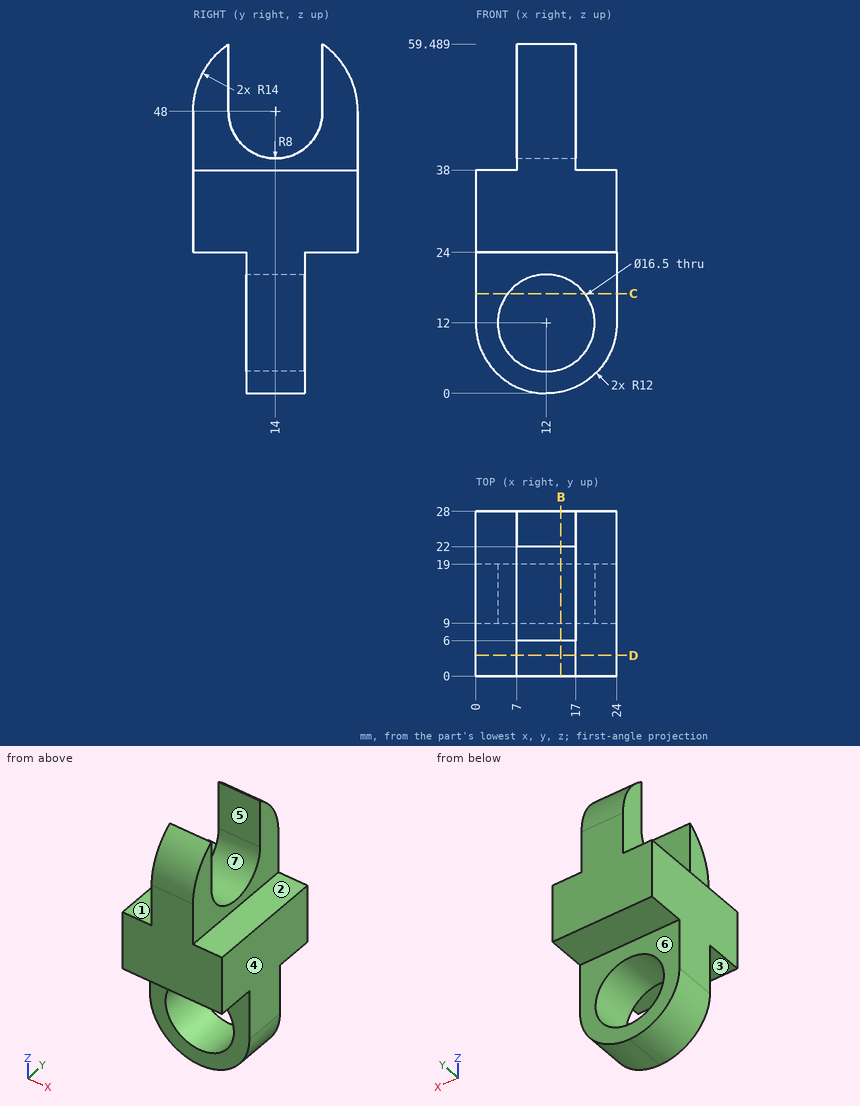
Geometry: see drawing. Coordinates: mm, zero at the bounding-box minimum. A direction names the side the tool comes from. Coordinates: 2 decimals unless noted, no trailing zeros. Loops run counter-clockwise (first coordinate to the right, second up) from the corner with the lowest first, then second, coordinate; pieces in that order, holes last. Notation, with made-up numbers: (-29, 50.25) -> (-10, 50.25) arc R13 cw to (-10, 54.25) -> close; hole circle Ø3 at (-9, 43.5). An arc over 180 degrees is marked (long way). Write item = value, one per line. Start each with the question number.
Item 1: Cut plane D-D, the plane y = 3.5. Return loops of the section in (x, z), plus the area to 3 significant figures.
Item 2: Reachability of the marked faces 1, 2 and 3 from +Z, -Z, +X, -X, +Y, -Y: full face, straight path, thin tool, end or side. Return the list, or none.
Item 3: First-contact query: P1, Ø5.5, axis at x = 3.5, y = 10.5, coming from the +Z side; P2, Ø10, axis at x = 3, y = 16.5, coming from the +Z side; P3, Ø10.5, axis at y = 20.5, z = 45.5, coming from the -X side; P4, Ø6.5, axis at y = 9.5, z = 50.5, coming from the +X side. Flat tips, straight axial feed; report the tip coordinate or a pass-through.
Item 4: Cut plane B-B, the plane x = 14.5. Return loops of the section in (y, z), plus the area to 3 significant figures.
Item 5: Cut plane C-C, the plane z = 17. Return loops of the section in (x, y).
Item 6: Material intervals for line 1 (X direction, y = 14.75, z = 12); line 2 (Z direction, x = 1, y = 23.25); line 3 (Y direction, x = 4.5, z = 5.5), sorted ascending.
Item 7: Mould query, pull axis Y, two halves, no side actions, for the marked faces 4, 5, 6 and 7. Classes: pulls with the +Y half, pulls with the -Y half, needs draft (parallel to the pull), parting line crosses it, or undercut.
Ans:
q1.outline = (0, 24) -> (24, 24) -> (24, 38) -> (17, 38) -> (17, 57.26) -> (7, 57.26) -> (7, 38) -> (0, 38) -> close
q1.area = 529 mm²
q2.face_1 = +Z, -X, +Y, -Y
q2.face_2 = +Z, +X, +Y, -Y
q2.face_3 = -Z, +X, -X, -Y
q3.P1 = 38
q3.P2 = 42.19
q3.P3 = 7
q3.P4 = through
q4.outline = (0, 24) -> (9, 24) -> (9, 19.86) -> (19, 19.86) -> (19, 24) -> (28, 24) -> (28, 48) arc R14 ccw to (22, 59.49) -> (22, 48) arc R8 cw to (6, 48) -> (6, 59.49) arc R14 ccw to (0, 48) -> close; (9, 0.26) -> (19, 0.26) -> (19, 4.14) -> (9, 4.14) -> close
q4.area = 748 mm²
q5.outline = (0, 9) -> (5.44, 9) -> (5.44, 19) -> (0, 19) -> close; (18.56, 9) -> (24, 9) -> (24, 19) -> (18.56, 19) -> close
q6.line_1 = 0 to 3.75, 20.25 to 24
q6.line_2 = 24 to 38
q6.line_3 = 9 to 19
q7.face_4 = needs draft
q7.face_5 = undercut
q7.face_6 = pulls with the +Y half
q7.face_7 = undercut
